```python
from build123d import *

# Parameters (mm, degrees)
SKETCH2_W           = 70
SKETCH2_H           = 60
BOSS_EXTRUDE1_DEPTH = 100
SKETCH3_R           = 7.5
CUT_EXTRUDE1_DEPTH  = 70
BOSS_EXTRUDE2_DEPTH = 70
FILLET1_R           = 10


with BuildPart() as part:
    # Sketch2 → Boss-Extrude1 (new body)
    with BuildSketch(Plane.XY):
        with Locations((0, 30)):
            Rectangle(SKETCH2_W, SKETCH2_H)
    extrude(amount=BOSS_EXTRUDE1_DEPTH)

    # Sketch3 → Cut-Extrude1 (cut)
    with BuildSketch(Plane.XY.offset(100)):
        with Locations((-17.5, 30)):
            Circle(SKETCH3_R)
        with Locations(Location((17.5, 30, 0), (0, 0, 180))):
            Circle(SKETCH3_R)
        with BuildLine():
            Line((35, 60), (-35, 60))
            Line((-35, 60), (-35, 30))
            ThreePointArc((-35, 30), (-17.5, 47.5), (0, 30))
            ThreePointArc((0, 30), (17.5, 47.5), (35, 30))
            Line((35, 30), (35, 60))
        make_face()
    extrude(amount=-CUT_EXTRUDE1_DEPTH, mode=Mode.SUBTRACT)

    # Sketch4 → Boss-Extrude2 (add)
    with BuildSketch(Plane.ZY.offset(35)):
        with BuildLine():
            Line((100, 0), (125, 0))
            Line((125, 0), (125, 10))
            ThreePointArc((125, 10), (135, 20), (145, 10))
            Line((145, 10), (145, 0))
            Line((145, 0), (170, 0))
            Line((170, 0), (170, 10))
            Line((170, 10), (152.5, 10))
            ThreePointArc((152.5, 10), (135, 27.5), (117.5, 10))
            Line((117.5, 10), (100, 10))
            Line((100, 10), (100, 0))
        make_face()
    extrude(amount=-BOSS_EXTRUDE2_DEPTH)

    # Fillet1
    fillet1_edges = [part.edges().sort_by_distance(p)[0] for p in [
        (-35, 60, 15),
        (35, 60, 15),
    ]]
    fillet(fillet1_edges, radius=FILLET1_R)


solid = part.part
```
Input: part model. Units: mm. Frame: model coordinates. A direction names the side the tool comes from. Round coordinates to 2 decimals unless told otherwise and drop trailing zeros. Write each loop counter-clockwise with the first axis right and the second up, starting at its lowest first coordinate (ties: lowest second). Pieces come first, ordered by that corner, then holes. Notation, with made-up numbers: M 7,26 L 30,26 A29 ccw 30,64 Z; hole C -25,14.25 d7. An arc over 180 degrees is marked long. Write each question's results on one line, items separated by ' | '.
Q1. Access query for faces 4 (the face through (0, 5, 145)), 5 (the face through (0, 52, 30)), 6 (the face through (-0.49, 27.496, 135.385)), 7 (the face through (32.15, 56.99, 15.21)), 8 (the face through (-23.452, 25.436, 65.49)). Directions: +Z, -Z, +X, -X, +Y, -Y. A direction counts if a zero-diameter tool reaches every point of the face in a straight line with its end or side. Return the directions, or none.
Results:
face 4: +X, -X, -Y | face 5: +Z, +Y | face 6: +X, -X, +Y | face 7: +Z, -Z, +X, +Y | face 8: none
Q2. Draft query along X for faces 1 (the face through (23.452, 34.564, 65.49)), 2 (the face through (-31.99, 57.15, 15.21)), 3 (the face through (0, 5, 170)). Return one class per face: released by +X, released by -X, zero draft, split by the parting line, or undercut.
Results:
face 1: undercut | face 2: released by -X | face 3: zero draft
Q3. Line query: line 1 along Z through (x, y) = (9, 4); line 2 along Y through (x, z) = (18, 33.5); line 3 along Z through (x, y) = (-14, 11). Output: solid intervals per line, ascending.
Results:
line 1: z = 0 to 125, 145 to 170 | line 2: y = 0 to 22.52, 37.48 to 47.49 | line 3: z = 0 to 100, 117.53 to 125.05, 144.95 to 152.47
Q4. Pin query (flat end, axial travel): P1, Ø9, axis at x = -4, z = 110, coming from the +Y side; P2, Ø16.5, axis at x = 18, y = 27, coming from the +Z side; P3, Ø9, axis at x = -10, y = 50, coming from the +Z side. Return the tip coordinate at first contact, or that it passes through.
Results:
P1: stops at y = 10 | P2: stops at z = 150.16 | P3: stops at z = 100
Q5. Section query A-A (x = -17.5). Return loops of the section in (y, z), and give its area (3 significant figures).
Results:
outline: M 0,0 L 60,0 L 60,30 L 47.5,30 L 47.5,100 L 37.5,100 L 37.5,30 L 22.5,30 L 22.5,100 L 10,100 L 10,117.5 A17.5 ccw 10,152.5 L 10,170 L 0,170 L 0,145 L 10,145 A10 cw 10,125 L 0,125 Z | area: 4,900 mm^2
Q6. Section query D-D (z = 106). Return loops of the section in (x, y).
Results:
outline: M -35,0 L 35,0 L 35,10 L -35,10 Z
Q7. Section query B-B (y = 12.5). Return loops of the section in (x, z).
Results:
outline: M -35,0 L 35,0 L 35,100 L -35,100 Z; M -35,117.68 L 35,117.68 L 35,125.32 L -35,125.32 Z; M -35,144.68 L 35,144.68 L 35,152.32 L -35,152.32 Z
Q8. Section query C-C (z = 74.5). Return loops of the section in (x, y), and give its area (3 significant figures).
Results:
outline: M -35,0 L 35,0 L 35,30 A17.5 ccw 0,30 A17.5 ccw -35,30 Z; hole C -17.5,30 d15; hole C 17.5,30 d15 | area: 2,710 mm^2
